The listing builds one solid part. Answer for the finished solid, in the listing's coordinates (mm). Face numbers are marked on the shaded views. Round coordinates to 2 decimals unless told otherwise and drop trailing zeros. Write each loop counter-clockwise with the first axis right and the second up, starting at its lowest first coordinate (ties: lowest second). Pieces come first, ordered by that corner, then holes.
from build123d import *

# Parameters (mm, degrees)
SKETCH1_R               = 5.5499
BOSS_EXTRUDE1_DEPTH     = 38.1
CUT_EXTRUDE1_DEPTH      = 17.78
SKETCH3_R               = 1.5875
CUT_EXTRUDE2_DEPTH      = 8.0499
CUT_EXTRUDE2_DEPTH_BACK = 5.0499
SKETCH4_R               = 5.5499
BOSS_EXTRUDE4_DEPTH     = 12.7
SKETCH6_R               = 5.5499
SKETCH6_R_2             = 5.12385248
CUT_EXTRUDE4_DEPTH      = 12.7


with BuildPart() as part:
    # Sketch1 → Boss-Extrude1 (new body)
    with BuildSketch(Plane.XY):
        Circle(SKETCH1_R)
    extrude(amount=BOSS_EXTRUDE1_DEPTH)

    # Sketch2 → Cut-Extrude1 (cut)
    with BuildSketch(Plane.XY.offset(38.1)):
        with BuildLine():
            Line((5.343350074, 1.5), (-5.343350074, 1.5))
            ThreePointArc((-5.343350074, 1.5), (-5.5499, 0), (-5.343350074, -1.5))
            Line((-5.343350074, -1.5), (5.343350074, -1.5))
            ThreePointArc((5.343350074, -1.5), (5.5499, 0), (5.343350074, 1.5))
        make_face()
    extrude(amount=-CUT_EXTRUDE1_DEPTH, mode=Mode.SUBTRACT)

    # Sketch3 → Cut-Extrude2 (cut, two sides)
    with BuildSketch(Plane(origin=(0, -1.5, 0), x_dir=(1, 0, 0), z_dir=(0, 1, 0))) as cut_extrude2_sk:
        with Locations((0, -34.036)):
            Circle(SKETCH3_R)
    extrude(amount=CUT_EXTRUDE2_DEPTH, mode=Mode.SUBTRACT)
    extrude(cut_extrude2_sk.sketch, amount=-CUT_EXTRUDE2_DEPTH_BACK, mode=Mode.SUBTRACT)

    # Sketch4 → Boss-Extrude4 (add)
    with BuildSketch(Plane.XY):
        Circle(SKETCH4_R)
    extrude(amount=-BOSS_EXTRUDE4_DEPTH)

    # Sketch6 → Cut-Extrude4 (cut)
    with BuildSketch(Plane.XY):
        Circle(SKETCH6_R)
        Circle(SKETCH6_R_2, mode=Mode.SUBTRACT)
    extrude(amount=CUT_EXTRUDE4_DEPTH, mode=Mode.SUBTRACT)


solid = part.part
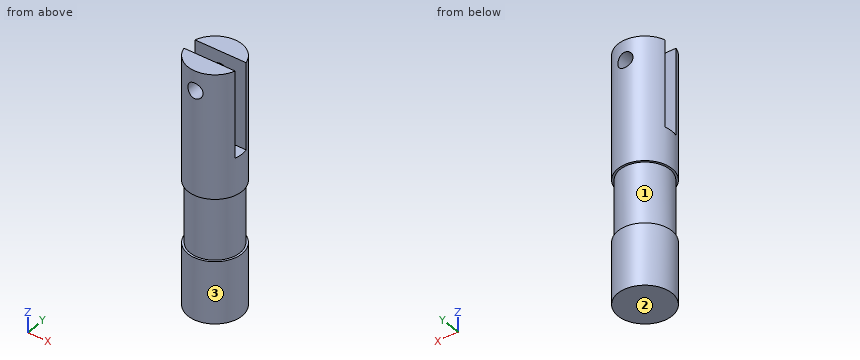
1. Section C-C on y = 0 is taken. Determine the outline of the cut face in (x, z), plus the area to 3 significant figures.
Geometry says:
outline: (-5.55, -12.7) - (5.55, -12.7) - (5.55, 0) - (5.12, 0) - (5.12, 12.7) - (5.55, 12.7) - (5.55, 20.32) - (-5.55, 20.32) - (-5.55, 12.7) - (-5.12, 12.7) - (-5.12, 0) - (-5.55, 0) - close
area: 356 mm2
2. Section B-B on z = 33 is taken. Determine the outline of the cut face in (x, y), plus the area to 3 significant figures.
Geometry says:
outline: (-5.34, -1.5) arc R5.55 ccw to (-1.2, -5.42) - (-1.2, -1.5) - close; (-5.34, 1.5) - (-1.2, 1.5) - (-1.2, 5.42) arc R5.55 ccw to start; (1.2, -5.42) arc R5.55 ccw to (5.34, -1.5) - (1.2, -1.5) - close; (1.2, 1.5) - (5.34, 1.5) arc R5.55 ccw to (1.2, 5.42) - close
area: 44.6 mm2
3. Section D-D on y = 2.25 is taken. Determine the outline of the cut face in (x, z) (1 decimal), plus the area to 3 significant figures.
Geometry says:
outline: (-5.1, -12.7) - (5.1, -12.7) - (5.1, 0) - (4.6, 0) - (4.6, 12.7) - (5.1, 12.7) - (5.1, 38.1) - (-5.1, 38.1) - (-5.1, 12.7) - (-4.6, 12.7) - (-4.6, 0) - (-5.1, 0) - close; hole circle Ø3.2 at (0, 34)
area: 496 mm2
4. Section A-A on x = 0 is taken. Determine the outline of the cut face in (y, z).
Geometry says:
outline: (-5.55, -12.7) - (5.55, -12.7) - (5.55, 0) - (5.12, 0) - (5.12, 12.7) - (5.55, 12.7) - (5.55, 32.45) - (1.5, 32.45) - (1.5, 20.32) - (-1.5, 20.32) - (-1.5, 32.45) - (-5.55, 32.45) - (-5.55, 12.7) - (-5.12, 12.7) - (-5.12, 0) - (-5.55, 0) - close; (-5.55, 35.62) - (-1.5, 35.62) - (-1.5, 38.1) - (-5.55, 38.1) - close; (1.5, 35.62) - (5.55, 35.62) - (5.55, 38.1) - (1.5, 38.1) - close
5. For a pull along Z with two mould halves and no side action, classify the marked faces 1, 2 and 3 as released by +Z, released by -Z, zero draft, split by the parting line, or undercut.
Geometry says:
face 1: undercut
face 2: released by -Z
face 3: zero draft
6. Given pin 1 (5.5 mm diameter, centred on x = 0, y = 1, fed in from +Z); pin 2 (4 mm diameter, centred on x = -0.5, z = 4, fed in from -Y); pin 3 (3 mm diameter, centred on x = -4, z = 13.5, fed in from -Y); pin 4 (2.5 mm diameter, centred on x = 0, z = 34.036, fed in from +Y), each flat-ended and moving along its own axis, determine where each tip first touches the part or whether it passes through.
Geometry says:
pin 1: stops at z = 38.1
pin 2: stops at y = -5.12
pin 3: stops at y = -4.95
pin 4: passes through
7. Straight lines are drawn through the part: line 1 along Z through (x, y) = (0, -2.5); line 2 along X through (y, z) = (-0.25, -6.5); line 3 along Y through (x, z) = (1, 23). For each, find the intervals that lie inside material, in ascending order.
Geometry says:
line 1: z = -12.7 to 32.45, 35.62 to 38.1
line 2: x = -5.54 to 5.54
line 3: y = -5.46 to -1.5, 1.5 to 5.46
